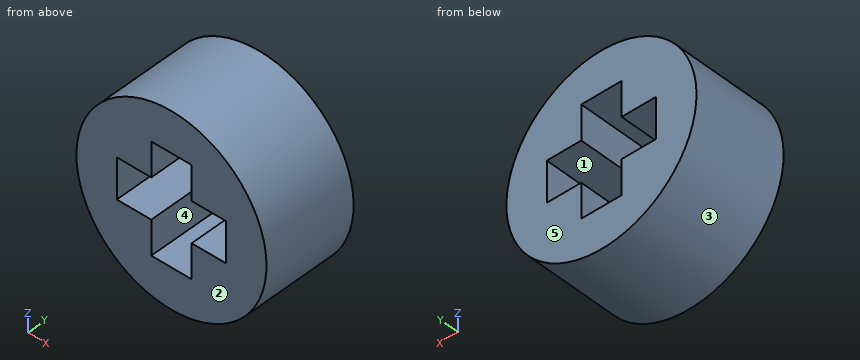
from build123d import *

# Parameters (mm, degrees)
SKETCH2_R           = 4
BOSS_EXTRUDE1_DEPTH = 4


with BuildPart() as part:
    # Sketch2 → Boss-Extrude1 (new body)
    with BuildSketch(Plane(origin=(0, 0, 0), x_dir=(1, 0, 0), z_dir=(0, 1, 0))):
        with Locations(Location((0, 0, 0), (0, 0, 270))):
            Circle(SKETCH2_R)
        Polygon((0.85, 0.85), (2.3, 0.85), (2.3, -0.85), (0.85, -0.85), (0.85, -2.3), (-0.85, -2.3), (-0.85, -0.85), (-2.3, -0.85), (-2.3, 0.85), (-0.85, 0.85), (-0.85, 2.3), (0.85, 2.3), align=None, mode=Mode.SUBTRACT)
    extrude(amount=BOSS_EXTRUDE1_DEPTH)


solid = part.part
Source: CAD feature listing. Evaluate the final solid. Frame: model axes, mm. Face numbers are marked on the shaded views. A direction names the side the tool comes from. Coordinates: 2 decimals unless noted, no trailing zeros. Loops run counter-clockwise (first coordinate to the right, second up) from the corner with the lowest first, then second, coordinate; pieces in that order, holes last. Notation, with made-up numbers: (24, 81) - (65, 81) arc R11 cw to (65, 88) - close; hole circle Ø7 at (26.25, -12.5). An arc over 180 degrees is marked (long way). One line per question, with ' | ' between items.
1) First-contact query: P1, Ø0.7, axis at y = 1.5, z = -1.5, coming from the +X side; P2, Ø1.6, axis at x = -1.5, y = 2, coming from the +Z side; P3, Ø0.7, axis at y = 2, z = -1.5, coming from the -X side. Flat tips, straight axial feed; report the tip coordinate or a pass-through.
Report:
P1: stops at x = 3.83 | P2: stops at z = 3.94 | P3: stops at x = -3.83
2) Line query: line 1 along X through (y, z) = (3.45, 0); line 2 along X through (y, z) = (2.2, -1.25); line 3 along Z through (x, y) = (-0.25, 1.65). Output: solid intervals per line, ascending.
Report:
line 1: x = -4 to -2.3, 2.3 to 4 | line 2: x = -3.8 to -0.85, 0.85 to 3.8 | line 3: z = -3.99 to -2.3, 2.3 to 3.99
3) Pull-direction query (X, two-part tool) for the marked faces 3, 4 and 5; classes: released by +X, released by -X, zero draft, split by the parting line, or undercut.
Report:
face 3: split by the parting line | face 4: undercut | face 5: zero draft
4) Set-up query: the marked faces 1 and 2. Return all of +Z, -Z, +X, -X, +Y, -Y with unobstructed straight access to the full face (end or side cutting, diameter ignored); none if empty.
Report:
face 1: +Y, -Y | face 2: +Z, -Z, +X, -X, -Y
5) Section C-C, the plane z = 0. Return loops of the section in (x, y).
Report:
outline: (-4, 0) - (-2.3, 0) - (-2.3, 4) - (-4, 4) - close; (2.3, 0) - (4, 0) - (4, 4) - (2.3, 4) - close
6) Section B-B, the plane x = 0. Return loops of the section in (y, z).
Report:
outline: (0, -4) - (4, -4) - (4, -2.3) - (0, -2.3) - close; (0, 2.3) - (4, 2.3) - (4, 4) - (0, 4) - close
7) Section D-D, the plane z = -2.75. Return loops of the section in (x, y), then the cut area to 3 significant figures.
Report:
outline: (-2.9, 0) - (2.9, 0) - (2.9, 4) - (-2.9, 4) - close | area: 23.2 mm²
8) Section A-A, the plane y = 1. Return loops of the section in (x, z), then the cut area to 3 significant figures.
Report:
outline: circle Ø8 at (0, 0); hole (-2.3, -0.85) - (-0.85, -0.85) - (-0.85, -2.3) - (0.85, -2.3) - (0.85, -0.85) - (2.3, -0.85) - (2.3, 0.85) - (0.85, 0.85) - (0.85, 2.3) - (-0.85, 2.3) - (-0.85, 0.85) - (-2.3, 0.85) - close | area: 37.5 mm²
